For this review, take the finished solid that the model builds, in its own axes (mm). Round coordinates to 2 decimals unless told otherwise and drop trailing zeros. Loops run counter-clockwise (first coordinate to the right, second up) from the corner with the lowest first, then second, coordinate; pieces in that order, holes last. Notation, with made-up numbers: M 52.25,22 L 70.25,22 A24 ccw 70.25,50 Z; hole C 75.25,-16 d11. An arc over 180 degrees is marked long. One line per question, with ' | ' between items. Start each with the question number.
1) Mouldability with a two-part tool opening along X and no side actions: class faces 1 (the face through (5.43, -286.37, 3.22)), 2 (the face through (56.23, -235.57, 3.22)), 3 (the face through (438.77, -286.67, 3.22)), 4 (the face through (387.97, -235.87, 3.22)) as pulls with the +X half, pulls with the -X half, needs draft (parallel to the pull), parting line crosses it, or undercut.
2) We need section B-B (z = 2.25). State how many separate pieces and enclosed holes the cut face has, and give its area (3 significant figures).
3) We need section C-C (x = 59.5). Give the boundary of the cut face in (y, z), and give its area (3 significant figures).
4) For probe 1 along X at (y, z) = (-50.8, 4.8); probe 2 along X at (y, z) = (-198.5, 5.75); probe 3 along X at (y, z) = (-88.5, 1.5), list the stretches that pass through material, from the lowest coordinate up. Write a range as from..to.
5) For pin 1 Ø8 at (x, y) = (19.05, -50.8) entering from -Z; pin 2 Ø4.5 at (x, y) = (401.64, -79.38) entering from -Z, all flat-tipped, find the tip position at first contact; note any pin that passes through.
6) We need section A-A (y = -252). Give the boundary of the cut face in (x, z), and give its area (3 significant figures).
```python
from build123d import *
from OCP.BRepFilletAPI import BRepFilletAPI_MakeChamfer

# Parameters (mm, degrees)
BOSS_EXTRUDE1_DEPTH             = 6.35
FILLET5_R                       = 19.05
FILLET6_R                       = 19.05
FILLET7_R                       = 19.05
FILLET8_R                       = 19.05
CUT_EXTRUDE1_DEPTH              = 532.923850283
CUT_EXTRUDE2_DEPTH              = 532.923850283
CHAMFER1_SIZE                   = 4.0894
CHAMFER1_SIZE2                  = 3.682112299
CHAMFER2_SIZE                   = 4.0894
CHAMFER2_SIZE2                  = 3.682112299
F_32_0_116_DIAMETER_HOLE1_D     = 2.9464
F_32_0_116_DIAMETER_HOLE1_DEPTH = 25.4
F_32_0_116_DIAMETER_HOLE1_TIP   = 0.885187864


with BuildPart() as part:
    # Sketch1 → Boss-Extrude1 (new body)
    with BuildSketch(Plane.XY):
        Polygon((0, 0), (0, -292.1), (444.5, -292.1), (444.5, 0), (393.7, 0), (393.7, -241.3), (50.8, -241.3), (50.8, 0), align=None)
    extrude(amount=BOSS_EXTRUDE1_DEPTH)

    # Fillet5
    fillet5_edges = [part.edges().sort_by_distance(p)[0] for p in [
        (0, -292.1, 3.175),
    ]]
    fillet(fillet5_edges, radius=FILLET5_R)

    # Fillet6
    fillet6_edges = [part.edges().sort_by_distance(p)[0] for p in [
        (444.5, -292.1, 3.175),
    ]]
    fillet(fillet6_edges, radius=FILLET6_R)

    # Fillet7
    fillet7_edges = [part.edges().sort_by_distance(p)[0] for p in [
        (50.8, -241.3, 3.175),
    ]]
    fillet(fillet7_edges, radius=FILLET7_R)

    # Fillet8
    fillet8_edges = [part.edges().sort_by_distance(p)[0] for p in [
        (393.7, -241.3, 3.175),
    ]]
    fillet(fillet8_edges, radius=FILLET8_R)

    # Sketch2 → Cut-Extrude1 (cut, through all)
    with BuildSketch(Plane.XY.offset(6.35)):
        with BuildLine():
            Line((22.1361, -260.35), (22.1361, -107.95))
            ThreePointArc((22.1361, -107.95), (25.4, -104.6861), (28.6639, -107.95))
            Line((28.6639, -107.95), (28.6639, -260.35))
            ThreePointArc((28.6639, -260.35), (25.4, -263.6139), (22.1361, -260.35))
        make_face()
    extrude(amount=-CUT_EXTRUDE1_DEPTH, mode=Mode.SUBTRACT)

    # Sketch4 → Cut-Extrude2 (cut, through all)
    with BuildSketch(Plane.XY.offset(6.35)):
        with BuildLine():
            Line((415.8361, -260.35), (415.8361, -107.95))
            ThreePointArc((415.8361, -107.95), (419.1, -104.6861), (422.3639, -107.95))
            Line((422.3639, -107.95), (422.3639, -260.35))
            ThreePointArc((422.3639, -260.35), (419.1, -263.6139), (415.8361, -260.35))
        make_face()
    extrude(amount=-CUT_EXTRUDE2_DEPTH, mode=Mode.SUBTRACT)

    # Sketch10 → CSK for 1/4 Flat Head Machine Screw2 (revolve, cut)
    with BuildSketch(Plane(origin=(19.05, -50.8, 0), x_dir=(0, 1, 0), z_dir=(1, 0, 0))):
        Polygon((0, 0), (0, 6.35), (3.3782, 6.35), (3.3782, 3.520932584), (6.4389, 0), align=None)
    revolve(axis=Axis((19.05, -50.8, -6.35), (0, 0, 1)), mode=Mode.SUBTRACT)

    # Chamfer1: one chamfer whose edges measure the first distance from different faces: ONE call of the kernel's chamfer builder (chamfer() names one face for all edges)
    chamfer1_edges_1 = [part.edges().sort_by_distance(p)[0] for p in [
        (419.1, -263.6139, 0),
    ]]
    chamfer1_side_1 = [part.faces().sort_by_distance(p)[0] for p in [
        (419.1, -263.6139, 3.175),
    ]]
    chamfer1_edges_2 = [part.edges().sort_by_distance(p)[0] for p in [
        (415.8361, -184.15, 0),
    ]]
    chamfer1_side_2 = [part.faces().sort_by_distance(p)[0] for p in [
        (415.8361, -184.15, 3.175),
    ]]
    chamfer1_edges_3 = [part.edges().sort_by_distance(p)[0] for p in [
        (419.1, -104.6861, 0),
    ]]
    chamfer1_side_3 = [part.faces().sort_by_distance(p)[0] for p in [
        (419.1, -104.6861, 3.175),
    ]]
    chamfer1_edges_4 = [part.edges().sort_by_distance(p)[0] for p in [
        (422.3639, -184.15, 0),
    ]]
    chamfer1_side_4 = [part.faces().sort_by_distance(p)[0] for p in [
        (422.3639, -184.15, 3.175),
    ]]
    chamfer1 = BRepFilletAPI_MakeChamfer(part.part.solid().wrapped)
    for e in chamfer1_edges_1:
        chamfer1.Add(CHAMFER1_SIZE, CHAMFER1_SIZE2, e.wrapped, chamfer1_side_1[0].wrapped)  # the first distance lies on this face
    for e in chamfer1_edges_2:
        chamfer1.Add(CHAMFER1_SIZE, CHAMFER1_SIZE2, e.wrapped, chamfer1_side_2[0].wrapped)  # the first distance lies on this face
    for e in chamfer1_edges_3:
        chamfer1.Add(CHAMFER1_SIZE, CHAMFER1_SIZE2, e.wrapped, chamfer1_side_3[0].wrapped)  # the first distance lies on this face
    for e in chamfer1_edges_4:
        chamfer1.Add(CHAMFER1_SIZE, CHAMFER1_SIZE2, e.wrapped, chamfer1_side_4[0].wrapped)  # the first distance lies on this face
    add(Compound.cast(chamfer1.Shape()), mode=Mode.REPLACE)

    # Chamfer2: one chamfer whose edges measure the first distance from different faces: ONE call of the kernel's chamfer builder (chamfer() names one face for all edges)
    chamfer2_edges_1 = [part.edges().sort_by_distance(p)[0] for p in [
        (25.4, -263.6139, 0),
    ]]
    chamfer2_side_1 = [part.faces().sort_by_distance(p)[0] for p in [
        (25.4, -263.6139, 3.175),
    ]]
    chamfer2_edges_2 = [part.edges().sort_by_distance(p)[0] for p in [
        (25.4, -104.6861, 0),
    ]]
    chamfer2_side_2 = [part.faces().sort_by_distance(p)[0] for p in [
        (25.4, -104.6861, 3.175),
    ]]
    chamfer2_edges_3 = [part.edges().sort_by_distance(p)[0] for p in [
        (28.6639, -184.15, 0),
    ]]
    chamfer2_side_3 = [part.faces().sort_by_distance(p)[0] for p in [
        (28.6639, -184.15, 3.175),
    ]]
    chamfer2_edges_4 = [part.edges().sort_by_distance(p)[0] for p in [
        (22.1361, -184.15, 0),
    ]]
    chamfer2_side_4 = [part.faces().sort_by_distance(p)[0] for p in [
        (22.1361, -184.15, 3.175),
    ]]
    chamfer2 = BRepFilletAPI_MakeChamfer(part.part.solid().wrapped)
    for e in chamfer2_edges_1:
        chamfer2.Add(CHAMFER2_SIZE, CHAMFER2_SIZE2, e.wrapped, chamfer2_side_1[0].wrapped)  # the first distance lies on this face
    for e in chamfer2_edges_2:
        chamfer2.Add(CHAMFER2_SIZE, CHAMFER2_SIZE2, e.wrapped, chamfer2_side_2[0].wrapped)  # the first distance lies on this face
    for e in chamfer2_edges_3:
        chamfer2.Add(CHAMFER2_SIZE, CHAMFER2_SIZE2, e.wrapped, chamfer2_side_3[0].wrapped)  # the first distance lies on this face
    for e in chamfer2_edges_4:
        chamfer2.Add(CHAMFER2_SIZE, CHAMFER2_SIZE2, e.wrapped, chamfer2_side_4[0].wrapped)  # the first distance lies on this face
    add(Compound.cast(chamfer2.Shape()), mode=Mode.REPLACE)

    # #32 (0.116) Diameter Hole1
    with Locations(Plane.XY.offset(6.35)):
        with Locations((401.6375, -73.025), (401.6375, -79.375)):
            Hole(F_32_0_116_DIAMETER_HOLE1_D / 2, depth=F_32_0_116_DIAMETER_HOLE1_DEPTH)
            with Locations((0, 0, -(F_32_0_116_DIAMETER_HOLE1_DEPTH + F_32_0_116_DIAMETER_HOLE1_TIP / 2))):  # 118° drill point
                Cone(0, F_32_0_116_DIAMETER_HOLE1_D / 2, F_32_0_116_DIAMETER_HOLE1_TIP, mode=Mode.SUBTRACT)


solid = part.part
```
Answers below:
1) face 1: pulls with the -X half | face 2: undercut | face 3: pulls with the +X half | face 4: undercut
2) separate pieces: 1 | enclosed holes: 5 | area: 43,900 mm^2
3) outline: M -292.1,0 L -238.24,0 L -238.24,6.35 L -292.1,6.35 Z | area: 342 mm^2
4) probe 1: 0..15.67, 22.43..50.8, 393.7..444.5 | probe 2: 0..22.14, 28.66..50.8, 393.7..415.84, 422.36..444.5 | probe 3: 0..50.8, 393.7..444.5
5) pin 1: z = 2.81 | pin 2: z = 0
6) outline: M 0,0 L 18.45,0 L 22.14,4.09 L 22.14,6.35 L 0,6.35 Z; M 28.66,4.09 L 32.35,0 L 412.15,0 L 415.84,4.09 L 415.84,6.35 L 28.66,6.35 Z; M 422.36,4.09 L 426.05,0 L 444.5,0 L 444.5,6.35 L 422.36,6.35 Z | area: 2,710 mm^2
